Read the model definition and answer for the solid it produces. Units are mm, in the model's axes. A direction names the side the tool comes from. Give positions to 0.01 mm unless a question says otherwise; leave off trailing zeros. Write each loop counter-clockwise with the first axis right and the second up, starting at its lowest first coordinate (ties: lowest second). Pieces come first, ordered by that corner, then holes. Notation, with made-up numbers: M 69,76 L 108,76 A24 cw 108,97 Z; hole C 11,-12.5 d9. An arc over 180 degrees is marked long. Answer as CSV lines item,"result". Start each with the question number.
```python
from build123d import *

# Parameters (mm, degrees)
SKETCH2_R           = 40
BOSS_EXTRUDE2_DEPTH = 190
SKETCH3_R           = 55
BOSS_EXTRUDE3_DEPTH = 55
SKETCH4_R           = 25
BOSS_EXTRUDE4_DEPTH = 7


with BuildPart() as part:
    # Sketch2 → Boss-Extrude2 (new body)
    with BuildSketch(Plane(origin=(0, 0, 0), x_dir=(1, 0, 0), z_dir=(0, 1, 0))):
        with Locations(Location((0, 0, 0), (0, 0, 270))):
            Circle(SKETCH2_R)
    extrude(amount=-BOSS_EXTRUDE2_DEPTH)

    # Sketch3 → Boss-Extrude3 (add, symmetric)
    with BuildSketch(Plane(origin=(0, 0, 0), x_dir=(0, 0, -1), z_dir=(1, 0, 0))):
        Circle(SKETCH3_R)
    extrude(amount=BOSS_EXTRUDE3_DEPTH, both=True)

    # Sketch4 → Boss-Extrude4 (add)
    with BuildSketch(Plane(origin=(30, 0, 0), x_dir=(0, 0, -1), z_dir=(1, 0, 0))):
        with BuildLine():
            Line((-18.395893308, -190), (18.395893308, -190))
            ThreePointArc((18.395893308, -190), (0, -254.775679831), (-18.395893308, -190))
        make_face()
        with Locations((0, -219.775679831)):
            Circle(SKETCH4_R, mode=Mode.SUBTRACT)
    boss_extrude4 = extrude(amount=-BOSS_EXTRUDE4_DEPTH)

    # Mirror1: Boss-Extrude4 across plane
    add(boss_extrude4.mirror(Plane(origin=(0, 0, 0), x_dir=(0, 0, 1), z_dir=(1, 0, 0))))


solid = part.part
```
1. Find section C-C on x = 27. Determine the outline of the cut face in (y, z).
2. For faces 3 (the face through (-39.05, -112.81, -8.67)), 4 (the face through (-55, 1, 1)), 5 (the face through (-30, -244, -8)), 6 (the face through (23, -244, -8)), 7 (the face through (30, -244, -8)), determine the directions among +Z, -Z, +X, -X, +Y, -Y from which every point of the face is accessible in a straight line to the end or side of a thin tool.
3. Given pin 1 (8 mm diameter, centred on x = 1.5, y = -34.5, fed in from +Z); pin 2 (2 mm diameter, centred on x = 21, z = -32.5, fed in from +Y); pin 3 (1.5 mm diameter, centred on x = -23.5, y = -210.5, fed in from +Z), each flat-ended and moving along its own axis, determine where each tip first touches the part or whether it passes through.
4. Find section A-A on z = 0. Determine the outline of the cut face in (x, y), then the cut area to 3 significant figures.
5. Determine the mould class of faces 1 (the face through (-23, -244, -8)), 2 (the face through (26.549, -194.988, 3.255)) for opening direction Y: +Y half, -Y half, draft (parallel to the pull), parting line (faces both ways), or undercut.
6. Find section B-B on y = -232.5. Determine the outline of the cut face in (x, z), then the cut area to 3 significant figures.
7. Find the intervals of material crossed by line 1 (Y direction, x = 24.75, z = 0); line 2 (Y direction, x = 29.5, z = -22.5); line 3 (Z direction, x = 1, y = -167), in increasing order. Write a range as [from, to].
8. Find section D-D on y = -98. Determine the outline of the cut face in (x, z), then the cut area to 3 significant figures.
Computed:
1,outline,"M -190,-29.51 L -46.41,-29.51 A55 ccw long -46.41,29.51 L -190,29.51 L -190,18.4 A35 ccw long -190,-18.4 Z; hole C -219.78,0 d50"
2,face 3,"none"
2,face 4,"+Z, -Z, -X, +Y, -Y"
2,face 5,"+Z, -Z, -X, -Y"
2,face 6,"+Z, -Z, -Y"
2,face 7,"+Z, -Z, +X, -Y"
3,pin 1,"stops at z = 45.77"
3,pin 2,"stops at y = 45.09"
3,pin 3,"stops at z = 33.95"
4,outline,"M -55,-55 L -40,-55 L -40,-190 L -30,-190 L -30,-194.78 L -23,-194.78 L -23,-190 L 23,-190 L 23,-194.78 L 30,-194.78 L 30,-190 L 40,-190 L 40,-55 L 55,-55 L 55,55 L -55,55 Z; M -30,-254.78 L -23,-254.78 L -23,-244.78 L -30,-244.78 Z; M 23,-254.78 L 30,-254.78 L 30,-244.78 L 23,-244.78 Z"
4,area,"23,100 mm^2"
5,face 1,"draft"
5,face 2,"undercut"
6,outline,"M -30,-32.61 L -23,-32.61 L -23,-21.52 L -30,-21.52 Z; M -30,21.52 L -23,21.52 L -23,32.61 L -30,32.61 Z; M 23,-32.61 L 30,-32.61 L 30,-21.52 L 23,-21.52 Z; M 23,21.52 L 30,21.52 L 30,32.61 L 23,32.61 Z"
6,area,"310 mm^2"
7,line 1,"y = [-254.78, -244.78], [-194.78, 55]"
7,line 2,"y = [-246.59, -230.67], [-208.88, -192.97], [-190, 50.19]"
7,line 3,"z = [-39.99, 39.99]"
8,outline,"C 0,0 d80"
8,area,"5,030 mm^2"
